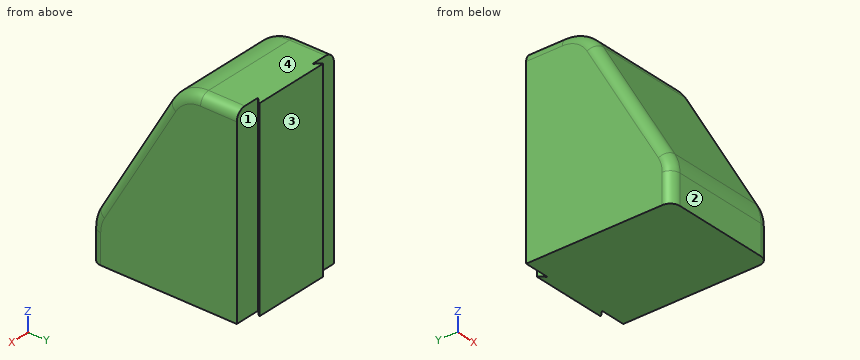
```python
from build123d import *

# Parameters (mm, degrees)
EXTRUDE1_DEPTH  = 152.4
EXTRUDE2_DEPTH  = 500
CHAMFER1_SIZE   = 1.796051224
CHAMFER1_SIZE_2 = 2.54
FILLET1_R       = 100
FILLET2_R       = 25.4


with BuildPart() as part:
    # Sketch1 → Extrude1 (new, symmetric)
    with BuildSketch(Plane(origin=(0, 0, 0), x_dir=(0, 0, -1), z_dir=(1, 0, 0))):
        Polygon((0, 0), (-500, 0), (-500, -152.4), (-104.05318539, -381), (0, -381), align=None)
    extrude(amount=EXTRUDE1_DEPTH, both=True)

    # Sketch2 → Extrude2 (add, through all)
    with BuildSketch(Plane(origin=(0, 0, 0), x_dir=(-1, 0, 0), z_dir=(0, 0, -1))):
        Polygon((-85.725, 0), (-101.6, 15.875), (101.6, 15.875), (85.725, 0), align=None)
    extrude(amount=-EXTRUDE2_DEPTH)

    # Chamfer1
    # the kernel refuses this chamfer: 2.54, 1.796051224 mm, written as the material it takes off along each edge
    with BuildSketch(Plane(origin=(-101.6, 15.875, -6.532074789), x_dir=(0.6660419652145836, -0.7459142715976788, 0), z_dir=(0, 0, 1)), Plane(origin=(101.6, 15.875, -6.532074789), x_dir=(-0.9984038297885897, 0.056478249472489896, 0), z_dir=(0, 0, 1))) as chamfer1_piece_1:
        Polygon((CHAMFER1_SIZE * 0.998403829907, CHAMFER1_SIZE * 0.0564782494792), (CHAMFER1_SIZE_2 * 0.666041965215, CHAMFER1_SIZE_2 * 0.745914271598), (0, 0), align=None)
    extrude(amount=513.064149579, mode=Mode.SUBTRACT)

    # Fillet1
    fillet1_edges = [part.edges().sort_by_distance(p)[0] for p in [
        (0, -381, 104.05318539),
        (0, -152.4, 500),
    ]]
    fillet(fillet1_edges, radius=FILLET1_R)

    # Fillet2
    fillet2_edges = [part.edges().sort_by_distance(p)[0] for p in [
        (-152.4, -381, 38.629133073),
        (-152.4, -377.592582629, 103.140170657),
        (-152.4, -274.435026919, 288.629133073),
        (-152.4, -144.664973081, 486.602540378),
        (152.4, -381, 38.629133073),
        (152.4, -377.592582629, 103.140170657),
        (152.4, -274.435026919, 288.629133073),
        (152.4, -144.664973081, 486.602540378),
        (-152.4, -47.332486541, 500),
        (152.4, -47.332486541, 500),
    ]]
    fillet(fillet2_edges, radius=FILLET2_R)


solid = part.part
```
Read the model definition and answer for the solid it produces. Units are mm, in the model's axes. Face numbers are marked on the shaded views. Give positions to 0.01 mm unless a question says otherwise; leave off trailing zeros. Order: outer loops, then holes, each group sorted by start corner. A loop starts at its lowest first (then second) coordinate and runs counter-clockwise, first axis right, second up. Notation, with made-up numbers: (4, 45.25) -> (57, 45.25) arc R22 ccw to (57, 61.25) -> close; hole circle Ø9 at (-39.75, 64.5). An arc over 180 degrees is marked (long way). One line per item, written item: value. Start each with the question number.
(1) For a pull along Y with two mould halves and no side action, classify the marked faces 1, 2, 3 and 4 as released by +Y, released by -Y, zero draft, split by the parting line, or undercut.
(2) Flat-ended cylindrical pins translate along their axes: P1, Ø3, axis at x = -12.5, z = 143, coming from the -Y side; P2, Ø2, axis at y = 14.5, z = 219, coming from the +X side; P3, Ø8, axis at x = -111.5, z = 97.5, coming from the -Y side. Find the tip coordinate at first contact, or state that the pin passes through.
(3) The part is cut by section A-A (x = -27). Determine the outline of the cut face in (y, z) (3 decimals).
(4) Straight lines are drawn through the part: L1, parallel to Y at x = 5.5, z = 81 (3 decimals); L2, parallel to Z at x = -37, y = -162.5; L3, parallel to Z at x = 120, y = -290. For each, find the intervals that lie inside material, in ascending order.
Taken from the geometry:
1. face 1: undercut
1. face 2: released by -Y
1. face 3: released by +Y
1. face 4: zero draft
2. P1: y = -359.38
2. P2: x = 99.8
2. P3: y = -379.67
3. outline: (-381, 0) -> (15.875, 0) -> (15.875, 500) -> (-94.665, 500) arc R100 ccw to (-181.268, 450) -> (-367.603, 127.258) arc R100 ccw to (-381, 77.258) -> close
4. L1: -380.93 to 15.875
4. L2: 0 to 473.47
4. L3: 0 to 261.67
